from build123d import *

# Parameters (mm, degrees)
F1_DEPTH = 30
F2_R     = 2.5
F3_DEPTH = 30


with BuildPart() as f1:
    # F0 (on Front) → F1 (new body)
    with BuildSketch(Plane.XZ):
        with BuildLine():
            ThreePointArc((7.5, 8), (6.914214, 9.414214), (5.5, 10))
            Line((5.5, 10), (-5.5, 10))
            ThreePointArc((-5.5, 10), (-6.914214, 9.414214), (-7.5, 8))
            Line((-7.5, 8), (-7.5, -8))
            ThreePointArc((-7.5, -8), (-6.914214, -9.414214), (-5.5, -10))
            Line((-5.5, -10), (5.5, -10))
            ThreePointArc((5.5, -10), (6.914214, -9.414214), (7.5, -8))
            Line((7.5, -8), (7.5, 8))
        make_face()
        with BuildLine():
            Line((-0.5, 5), (0.5, 5))
            ThreePointArc((0.5, 5), (1.914214, 4.414214), (2.5, 3))
            Line((2.5, 3), (2.5, -3))
            ThreePointArc((2.5, -3), (1.914214, -4.414214), (0.5, -5))
            Line((0.5, -5), (-0.5, -5))
            ThreePointArc((-0.5, -5), (-1.914214, -4.414214), (-2.5, -3))
            Line((-2.5, -3), (-2.5, 3))
            ThreePointArc((-2.5, 3), (-1.914214, 4.414214), (-0.5, 5))
        make_face(mode=Mode.SUBTRACT)
    extrude(amount=F1_DEPTH)

    # F2 (on Right) → F3 (cut)
    with BuildSketch(Plane.YZ):
        with Locations((-15, 0)):
            Circle(F2_R)
    extrude(amount=-F3_DEPTH, mode=Mode.SUBTRACT)


solid = f1.part
Can you work these out from the model? Positions are in its coordinate system, mm. A direction names the side the tool comes from. Coordinates: 2 decimals unless noted, no trailing zeros. Write each loop counter-clockwise with the first axis right and the second up, starting at its lowest first coordinate (ties: lowest second). Pieces come first, ordered by that corner, then holes. Notation, with made-up numbers: (76.5, 74) - (128.5, 74) arc R11 cw to (128.5, 90) - close; hole circle Ø4 at (40.5, -0.5). An arc over 180 degrees is marked (long way). Return JSON: item names as keys, results as strings. Group by question number.
Item 1: If we section it at C-C (y = -15): Write out the boundary of the cut face in (x, z), then the cut area to 3 significant figures.
Item 2: If we section it at D-D (z = 3.5): Write out the boundary of the cut face in (x, y), then the cut area to 3 significant figures.
Item 3: Please list where these lines run through material, in increasing order: probe 1 along Z at (x, y) = (-4.7, -15); probe 2 along X at (y, z) = (-25.5, -1.5); probe 3 along Z at (x, y) = (0.25, -19.25).
Item 4: Which directions (+Z, -Z, +X, -X, +Y, -Y) give clear straight access to the entire face, cutting with the end or side of a thin tool? Please do faces 5 (the face through (0, -15, -10)), 6 (the face through (-1.9, -14.79, -4.43)).
Item 5: If we section it at A-A (z = -2): Write out the boundary of the cut face in (x, y), then the cut area to 3 significant figures.
Item 6: If we section it at B-B (y = -8.5): Write out the boundary of the cut face in (x, z), then the cut area to 3 significant figures.
Item 7: We'd pull the mould along X, two halves only. Please class faces 1 (the face through (-2.5, -14.8, -2.7)), 2 (the face through (-7.5, -11, 0)), 3 (the face through (1.93, -14.79, -4.4)), 4 (the face through (-5, -17.5, 0.1)): pulls with the +X half, pulls with the -X half, needs draft (parallel to the pull), parting line crosses it, or undercut.
Item 8: I'm going to push flat-ended pins straight in: pin 1 Ø4.5 at (y, z) = (-15, 0) entering from -X; pin 2 Ø3 at (x, z) = (-4.5, 4.5) entering from +Y. Where does each tip first touch, or does it pass through?
Return value:
{
 "1": {"outline": "(-7.5, -8) arc R2 ccw to (-5.5, -10) - (5.5, -10) arc R2 ccw to (7.5, -8) - (7.5, 8) arc R2 ccw to (5.5, 10) - (-5.5, 10) arc R2 ccw to (-7.5, 8) - (-7.5, 2.5) - (-2.5, 2.5) - (-2.5, 3) arc R2 cw to (-0.5, 5) - (0.5, 5) arc R2 cw to (2.5, 3) - (2.5, -3) arc R2 cw to (0.5, -5) - (-0.5, -5) arc R2 cw to (-2.5, -3) - (-2.5, -2.5) - (-7.5, -2.5) - close", "area": "225 mm^2"},
 "2": {"outline": "(-7.5, -30) - (-2.44, -30) - (-2.44, 0) - (-7.5, 0) - close; (2.44, -30) - (7.5, -30) - (7.5, 0) - (2.44, 0) - close", "area": "304 mm^2"},
 "3": {"probe 1": "z = -10 to -2.5, 2.5 to 10", "probe 2": "x = -7.5 to -2.5, 2.5 to 7.5", "probe 3": "z = -10 to -5, 5 to 10"},
 "4": {"face 5": "-Z, +X, -X, +Y, -Y", "face 6": "+Y, -Y"},
 "5": {"outline": "(-7.5, -30) - (-2.5, -30) - (-2.5, -16.5) - (-7.5, -16.5) - close; (-7.5, -13.5) - (-2.5, -13.5) - (-2.5, 0) - (-7.5, 0) - close; (2.5, -30) - (7.5, -30) - (7.5, 0) - (2.5, 0) - close", "area": "285 mm^2"},
 "6": {"outline": "(-7.5, -8) arc R2 ccw to (-5.5, -10) - (5.5, -10) arc R2 ccw to (7.5, -8) - (7.5, 8) arc R2 ccw to (5.5, 10) - (-5.5, 10) arc R2 ccw to (-7.5, 8) - close; hole (-2.5, -3) arc R2 ccw to (-0.5, -5) - (0.5, -5) arc R2 ccw to (2.5, -3) - (2.5, 3) arc R2 ccw to (0.5, 5) - (-0.5, 5) arc R2 ccw to (-2.5, 3) - close", "area": "250 mm^2"},
 "7": {"face 1": "undercut", "face 2": "pulls with the -X half", "face 3": "undercut", "face 4": "needs draft"},
 "8": {"pin 1": "stops at x = 2.5", "pin 2": "stops at y = 0"}
}
